Can you work these out from the model? Positions are in its coordinate system, mm. A direction names the side the tool comes from. Coordinates: 2 decimals unless noted, no trailing zeros. Loops run counter-clockwise (first coordinate to the right, second up) from the corner with the lowest first, then second, coordinate; pieces in that order, holes last. Notation, with made-up numbers: M -27.5,-33 L -21.5,-33 A20 ccw -21.5,-18 Z; hole C 59,54 d8. An arc over 180 degrees is marked long. Return JSON: item names as keys, results as strings. Group by question number.
```python
from build123d import *

# Parameters (mm, degrees)
PAD_DEPTH        = 7
HOLE_D           = 15
HOLE_CBORE_D     = 22
HOLE_CBORE_DEPTH = 6
FILLET_R         = 1


with BuildPart() as part:
    # Sketch002 → Pad (new body)
    with BuildSketch(Plane.XY):
        with BuildLine():
            ThreePointArc((0.652174, 71.252227), (14.996453, 86.564207), (0, 101.238043))
            ThreePointArc((0, 101.238043), (-26.162951, 90.400994), (-37, 64.238043))
            Line((-37, 64.238043), (-37, 0))
            ThreePointArc((-37, 0), (-22, -15), (-7, 0))
            Line((-7, 0), (-7, 63.259792))
            ThreePointArc((0.652174, 71.252227), (-4.778521, 68.792305), (-7, 63.259792))
        make_face()
    extrude(amount=PAD_DEPTH)

    # Hole (through all)
    with Locations(Plane(origin=(0, 0, 0), x_dir=(1, 0, 0), z_dir=(0, 0, -1))):
        with Locations((0, -86.238043), (-22, 0)):
            CounterBoreHole(HOLE_D / 2, HOLE_CBORE_D / 2, HOLE_CBORE_DEPTH)

    # Fillet
    fillet_edges = [part.edges().sort_by_distance(p)[0] for p in [
        (-37, 32.119021, 0),
        (-37, 32.119021, 7),
    ]]
    fillet(fillet_edges, radius=FILLET_R)


solid = part.part
```
1) Suppose I cut it at A-A, the plane y = 13.5. List the corners of the cut face in (x, z) for me.
2) For pin 1 (19.5 mm diameter, centred on x = -22, y = 0, fed in from -Z); pin 2 (13 mm diameter, centred on x = 0, y = 86.24, fed in from +Z); pin 3 (4 mm diameter, centred on x = -9.5, z = 5.5, fed in from +Y); pin 4 (1.5 mm diameter, centred on y = 51.5, z = 1, fed in from +X), each with a flat end and sliding along its axis, tell me the tip position at first contact or that it passes through.
3) Suppose I cut it at B-B, the plane z = 3.5. List the corners of the cut face in (x, y) for me.
4) For faces 4 (the face through (-7, 31, 3)), 5 (the face through (-37, 33, 3)), 6 (the face through (7.2, 83.6, 6)), which set-ups out of +Z, -Z, +X, -X, +Y, -Y let a thin tool reach every point of the face, with its end or its side?
5) If I drill on line 1 (Z direction, x = -14, y = 5); line 2 (X direction, y = 41.5, z = 2.25); line 3 (Y direction, x = 0, z = 4.3), over which ranges is the centre line in solid material (lowest first)? Write a range as from..to.
6) If we mould it in two halves opening along Y, with no side actions, what happens to faces 1 (the face through (-17, 44, 7)), 2 (the face through (-25.87, 90.69, 3.46)), 3 (the face through (-11.839, 4.213, 2.958))? For each: +Y half, -Y half, draft (parallel to the pull), parting line (faces both ways), or undercut.
Returned:
{
 "1": {"outline": "M -37,1 A1 ccw -36,0 L -8,0 A1 ccw -7,1 L -7,6 A1 ccw -8,7 L -36,7 A1 ccw -37,6 Z"},
 "2": {"pin 1": "stops at z = 6", "pin 2": "passes through", "pin 3": "stops at y = 100.47", "pin 4": "stops at x = -7"},
 "3": {"outline": "M -37,0 A15 ccw -7,0 L -7,63.26 A8 cw 0.65,71.25 A15 ccw 0,101.24 A37 ccw -37,64.24 Z; hole C -22,0 d22; hole C 0,86.24 d22"},
 "4": {"face 4": "+Z, -Z, +X, -Y", "face 5": "+Z, -Z, -X, +Y, -Y", "face 6": "-Z"},
 "5": {"line 1": "z = 6..7", "line 2": "x = -37..-7", "line 3": "y = 71.2..75.24, 97.24..101.24"},
 "6": {"face 1": "draft", "face 2": "+Y half", "face 3": "undercut"}
}
